The listing builds one solid part. Answer for the finished solid, in the listing's coordinates (mm). Round coordinates to 2 decimals unless told otherwise and drop trailing zeros. Loops run counter-clockwise (first coordinate to the right, second up) from the corner with the lowest first, then second, coordinate; pieces in that order, holes last. Notation, with made-up numbers: (28, -29.5) - (72, -29.5) arc R19 ccw to (72, -9.5) - close; hole circle Ø8 at (-17.5, 52). An arc over 180 degrees is marked (long way). One line per item, written item: value.
```python
from build123d import *

# Parameters (mm, degrees)
BOSS_EXTRUDE1_DEPTH             = 6.35
LPATTERN1_COUNT                 = 5
LPATTERN1_PITCH                 = 2
SKETCH4_W                       = 10
SKETCH4_H                       = 6
BOSS_EXTRUDE3_DEPTH             = 6
FILLET1_R                       = 0.25
M5X0_8_TAPPED_HOLE1_D           = 4.2
M5X0_8_TAPPED_HOLE1_CSINK_D     = 5.05
M5X0_8_TAPPED_HOLE1_CSINK_ANGLE = 90


with BuildPart() as part:
    # Sketch1 → Boss-Extrude1 (new, symmetric)
    with BuildSketch(Plane.XY):
        with BuildLine():
            Line((0, 0), (0, -0.254))
            Line((0, -0.254), (0.259824575, -0.254))
            ThreePointArc((0.259824575, -0.254), (0.358731646, -0.291228588), (0.408543109, -0.384434783))
            ThreePointArc((0.408543109, -0.384434783), (0.442388286, -0.542062154), (0.501123596, -0.692202247))
            ThreePointArc((0.501123596, -0.692202247), (0.705850588, -0.919639059), (1, -1.004))
            Line((1, -1.004), (1, 0))
            Line((1, 0), (1, 0.516))
            Line((1, 0.516), (0, 0.516))
            Line((0, 0.516), (0, 0))
        make_face()
    extrude(amount=BOSS_EXTRUDE1_DEPTH, both=True)

    # Mirror1: part across plane


with BuildPart() as part_1:
    add(part.part)
    add(part.part.mirror(Plane(origin=(1, 0.516, 6.35), x_dir=(0, 0, 1), z_dir=(-1, 0, 0))))


with BuildPart() as lpattern1_1:
    # LPattern1: pattern copy
    add(part_1.part.moved(Location(Vector(-1, 0, 0) * (1 * LPATTERN1_PITCH))))


with BuildPart() as lpattern1_2:
    # LPattern1: pattern copy
    add(part_1.part.moved(Location(Vector(-1, 0, 0) * (2 * LPATTERN1_PITCH))))


with BuildPart() as lpattern1_3:
    # LPattern1: pattern copy
    add(part_1.part.moved(Location(Vector(-1, 0, 0) * (3 * LPATTERN1_PITCH))))


with BuildPart() as lpattern1_4:
    # LPattern1: pattern copy
    add(part_1.part.moved(Location(Vector(-1, 0, 0) * (4 * LPATTERN1_PITCH))))


with BuildPart() as lpattern1_1_1:
    add(lpattern1_1.part)

    # Combine1: union LPattern1_4, part, LPattern1_3, LPattern1_2
    add(lpattern1_4.part)
    add(part_1.part)
    add(lpattern1_3.part)
    add(lpattern1_2.part)


with BuildPart() as body_2:
    # Sketch4 → Boss-Extrude3 (new, symmetric)
    with BuildSketch(Plane.XY):
        with Locations((-3, -2.484)):
            Rectangle(SKETCH4_W, SKETCH4_H)
    extrude(amount=BOSS_EXTRUDE3_DEPTH, both=True)

    # Combine2: cut LPattern1_1
    add(lpattern1_1_1.part, mode=Mode.SUBTRACT)

    # Mirror2: body 2 across plane


with BuildPart() as body_2_1:
    add(body_2.part)
    add(body_2.part.mirror(Plane(origin=(2, -5.484, 6), x_dir=(0, 0, 1), z_dir=(0, 1, 0))))

    # Fillet1
    fillet1_edges = [body_2_1.edges().sort_by_distance(p)[0] for p in [
        (2, -10.714, 0),
        (-8, -10.714, 0),
        (-8, -0.254, 0),
        (2, -0.254, 0),
    ]]
    fillet(fillet1_edges, radius=FILLET1_R)

    # M5x0.8 Tapped Hole1 (through all)
    with Locations(Plane.ZY.offset(8)):
        with Locations((0, -5.484)):
            CounterSinkHole(M5X0_8_TAPPED_HOLE1_D / 2, M5X0_8_TAPPED_HOLE1_CSINK_D / 2, counter_sink_angle=M5X0_8_TAPPED_HOLE1_CSINK_ANGLE)


solid = body_2_1.part
```
1) For a pull along Y with two mould halves and no side action, classify faces 1 (the cylindrical face through (-2.72, -3.713, -1.129)), 2 (the flat face through (2, -8, 0)) as released by +Y, released by -Y, zero draft, split by the parting line, or undercut.
Final values:
face 1: undercut
face 2: zero draft
2) Consider L1, parallel to Y at x = -0.25, z = 0; L2, parallel to Y at x = -0.5, z = 0; L3, parallel to X at y = -10.5, z = 5.25. Determine where each line is inside the solid, lowest interval first.
Final values:
L1: -10.71 to -7.58, -3.38 to -0.25
L2: -10.28 to -7.58, -3.38 to -0.69
L3: -8 to -7.58, -6.42 to -5.58, -4.42 to -3.58, -2.42 to -1.58, -0.42 to 0.42, 1.58 to 2
3) A cutting plane is placed at A-A on x = 1.25. Give the vertices of the cut face in (y, z).
Final values:
outline: (-10.02, -6) - (-0.94, -6) - (-0.94, 6) - (-10.02, 6) - close; hole circle Ø4.2 at (-5.48, 0)
